from build123d import *

# Parameters (mm, degrees)
F0_R          = 16.51
F1_DEPTH      = 152.4
F1_DEPTH_BACK = 152.4
F2_R          = 16.51
F3_DEPTH      = 152.4
F5_R          = 16.51
F6_DEPTH      = 152.4
F7_R          = 15.875
F8_DEPTH      = 304.801
F9_R          = 15.875
F10_DEPTH     = 152.41
F11_R         = 15.875
F12_DEPTH     = 152.41


with BuildPart() as f1:
    # F0 (on Front) → F1 (new body, two sides)
    with BuildSketch(Plane.XZ) as f1_sk:
        Circle(F0_R)
    extrude(amount=F1_DEPTH)
    extrude(f1_sk.sketch, amount=-F1_DEPTH_BACK)

    # F2 (on Right) → F3 (join)
    with BuildSketch(Plane.YZ):
        Circle(F2_R)
    extrude(amount=F3_DEPTH)

    # F5 (on face) → F6 (join)
    with BuildSketch(Plane(origin=(0, 0, 0), x_dir=(0, 1, 0), z_dir=(0.7071067812, 0, 0.7071067812))):
        Circle(F5_R)
    extrude(amount=-F6_DEPTH)

    # F7 (on face) → F8 (cut, through all)
    with BuildSketch(Plane.XZ.offset(152.4)):
        Circle(F7_R)
    extrude(amount=-F8_DEPTH, mode=Mode.SUBTRACT)

    # F9 (on face) → F10 (cut, up to face)
    with BuildSketch(Plane.YZ.offset(152.4)):
        Circle(F9_R)
    extrude(amount=-F10_DEPTH, mode=Mode.SUBTRACT)

    # F11 (on face) → F12 (cut, up to face)
    with BuildSketch(Plane(origin=(-107.7630734528, 0, -107.7630734528), x_dir=(0, -1, 0), z_dir=(-0.7071067812, 0, -0.7071067812))):
        Circle(F11_R)
    extrude(amount=-F12_DEPTH, mode=Mode.SUBTRACT)


solid = f1.part
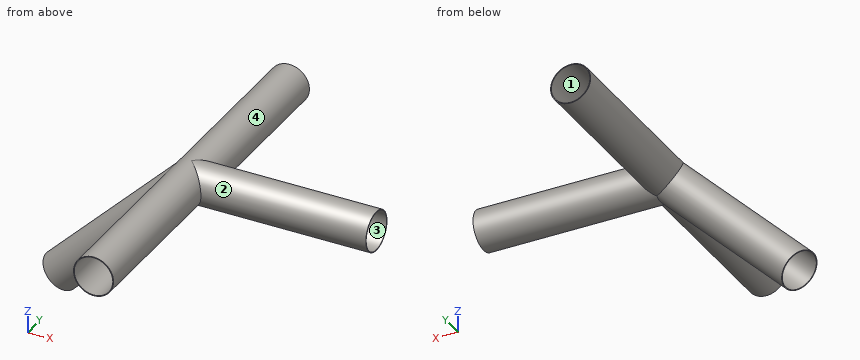
Source: CAD feature listing. Evaluate the final solid. Frame: model axes, mm. Face numbers are marked on the shaded views. A direction names the side the tool comes from. Give positions to 0.01 mm unless a question says otherwise; leave off trailing zeros. Loops run counter-clockwise (first coordinate to the right, second up) from the corner with the lowest first, then second, coordinate; pieces in that order, holes last. Notation, with made-up numbers: (-21.5, 4.25) -> (6.5, 4.25) arc R20 cw to (6.5, 33.25) -> close; hole circle Ø11 at (-6, 87). An arc over 180 degrees is marked (long way). Use a Markdown table: item, result. Add a question column.
1) First-contact query: pin 1 (8 mm diameter, centred on y = 92, z = 1.5, fed in from -X); pin 2 (1 mm diameter, centred on x = 75.5, y = -3.5, fed in from +Z); pin 3 (10 mm diameter, centred on y = -74, z = 2.5, fed in from +X). Flat tips, straight axial feed; report the tip coordinate or a pass-through.
2) Reachability of the marked faces 3 and 4 from +Z, -Z, +X, -X, +Y, -Y: full face, straight path, thin tool, end or side. Return the list, or none.
3) Section query C-C, the plane z = 0. Count the separate pieces of the cut face and the enclosed holes in it, then the cut area to 3 significant figures.
4) Pull-direction query (Z, two-part tool) for the marked faces 1 and 2; classes: +Z half, -Z half, draft (parallel to the pull), parting line (faces both ways), or undercut.
5) Line query: line 1 along Z through (x, y) = (0, -84) (3 decimals). Output: solid intervals per line, ascending. Write a range as [from, to].
6) Section query A-A, the plane x = 38.5. Return the cut outline in (y, z) (3 decimals), then the cut area to 3 significant figures.
Numbers:
| question | item | result |
|---|---|---|
| 1 | pin 1 | stops at x = -16.51 |
| 1 | pin 2 | stops at z = 16.24 |
| 1 | pin 3 | stops at x = 16.51 |
| 2 | face 3 | +X |
| 2 | face 4 | none |
| 3 | separate pieces | 3 |
| 3 | enclosed holes | 0 |
| 3 | area | 548 mm2 |
| 4 | face 1 | undercut |
| 4 | face 2 | parting line |
| 5 | line 1 | z = [-16.51, -15.875], [15.875, 16.51] |
| 6 | outline | circle Ø33.02 at (0, 0); hole circle Ø31.75 at (0, 0) |
| 6 | area | 64.6 mm2 |
